Verification items for the finished model (mm, model axes). A direction names the side the tool comes from. Give positions to 0.01 mm unless a question says otherwise; leave off trailing zeros. Loops run counter-clockwise (first coordinate to the right, second up) from the corner with the lowest first, then second, coordinate; pieces in that order, holes last. Notation, with made-up numbers: (77, -23.75) -> (108, -23.75) arc R33 cw to (108, 6.25) -> close; hole circle Ø5 at (-40, 23.5). An arc over 180 degrees is marked (long way). Answer in a Markdown table with one row per item. Add a question column.
Q1. Gauge pin test, flat ends, axial feed: P1, Ø1, axis at x = -440.5, y = -16, coming from the -Z side; P2, Ø4, axis at x = -154.5, y = -15.5, coming from the +Z side. Record the tip position at first contact, or that the pin passes through.
Q2. Material ranges on probe 1 along X at (y, z) = (-17.25, 167) (3 decimals); probe 2 along Z at (x, y) = (-696.5, -17.25); probe 3 along X at (y, z) = (-10.5, 149), recorded low to high.
Q3. Section check D-D on z = 49.5. Enter the section's corners in (x, y).
Q4. Section check A-A on z = 178. Enter the section's corners in (x, y) (3 decimals), and give its area (3 significant figures).
Q5. Section check B-B on y = -15.25. Enter the section's corners in (x, z) (3 decimals).
Q6. Release check for a two-part mould opening along X. For faces 1 (the face through (-422, 0, 103)), 2 (the face through (-92.968, -9.392, 147.338)), 3 (the face through (-831.85, -9, 103)) record: pulls with the +X half, pulls with the -X half, needs draft (parallel to the pull), parting line crosses it, or undercut.
Q7. Set-up check for faces 4 (the face through (-746.125, -9, 22)), 5 (the face through (-793, -9, 0)), 6 (the face through (-412, -9, 139.7)): record each of +Z, -Z, +X, -X, +Y, -Y from which the full face is reachable in a straight line by a thin tool's end or side.
Q8. Section check C-C on x = -547. Enter the section's corners in (y, z), and give its area (3 significant figures).
```python
from build123d import *

# Parameters (mm, degrees)
F1_DEPTH = 19.05


with BuildPart() as f1:
    # F0 (on Front) → F1 (new body)
    with BuildSketch(Plane.XZ):
        with BuildLine():
            Line((-752.475, 203.2), (-831.85, 203.2))
            Line((-831.85, 203.2), (-831.85, 0))
            Line((-831.85, 0), (-752.475, 0))
            ThreePointArc((-752.475, 0), (-747.984872, 1.859872), (-746.125, 6.35))
            Line((-746.125, 6.35), (-746.125, 38.1))
            ThreePointArc((-746.125, 38.1), (-738.685512, 56.060512), (-720.725, 63.5))
            Line((-720.725, 63.5), (-111.125, 63.5))
            ThreePointArc((-111.125, 63.5), (-93.164488, 56.060512), (-85.725, 38.1))
            Line((-85.725, 38.1), (-85.725, 6.35))
            ThreePointArc((-85.725, 6.35), (-83.865128, 1.859872), (-79.375, 0))
            Line((-79.375, 0), (0, 0))
            Line((0, 0), (0, 203.2))
            Line((0, 203.2), (-79.375, 203.2))
            ThreePointArc((-79.375, 203.2), (-83.865128, 201.340128), (-85.725, 196.85))
            Line((-85.725, 196.85), (-85.725, 165.1))
            ThreePointArc((-85.725, 165.1), (-93.164488, 147.139488), (-111.125, 139.7))
            Line((-111.125, 139.7), (-720.725, 139.7))
            ThreePointArc((-720.725, 139.7), (-738.685512, 147.139488), (-746.125, 165.1))
            Line((-746.125, 165.1), (-746.125, 196.85))
            ThreePointArc((-746.125, 196.85), (-747.984872, 201.340128), (-752.475, 203.2))
        make_face()
    extrude(amount=F1_DEPTH)


solid = f1.part
```
Taken from the geometry:
| question | item | result |
|---|---|---|
| 1 | P1 | stops at z = 63.5 |
| 1 | P2 | stops at z = 139.7 |
| 2 | probe 1 | x = -831.85 to -746.125, -85.725 to 0 |
| 2 | probe 2 | z = 63.5 to 139.7 |
| 2 | probe 3 | x = -831.85 to -740.37, -91.48 to 0 |
| 3 | outline | (-831.85, -19.05) -> (-743.42, -19.05) -> (-743.42, 0) -> (-831.85, 0) -> close; (-88.43, -19.05) -> (0, -19.05) -> (0, 0) -> (-88.43, 0) -> close |
| 4 | outline | (-831.85, -19.05) -> (-746.125, -19.05) -> (-746.125, 0) -> (-831.85, 0) -> close; (-85.725, -19.05) -> (0, -19.05) -> (0, 0) -> (-85.725, 0) -> close |
| 4 | area | 3,270 mm² |
| 5 | outline | (-831.85, 0) -> (-752.475, 0) arc R6.35 ccw to (-746.125, 6.35) -> (-746.125, 38.1) arc R25.4 cw to (-720.725, 63.5) -> (-111.125, 63.5) arc R25.4 cw to (-85.725, 38.1) -> (-85.725, 6.35) arc R6.35 ccw to (-79.375, 0) -> (0, 0) -> (0, 203.2) -> (-79.375, 203.2) arc R6.35 ccw to (-85.725, 196.85) -> (-85.725, 165.1) arc R25.4 cw to (-111.125, 139.7) -> (-720.725, 139.7) arc R25.4 cw to (-746.125, 165.1) -> (-746.125, 196.85) arc R6.35 ccw to (-752.475, 203.2) -> (-831.85, 203.2) -> close |
| 6 | face 1 | needs draft |
| 6 | face 2 | undercut |
| 6 | face 3 | pulls with the -X half |
| 7 | face 4 | -Z, +Y, -Y |
| 7 | face 5 | -Z, +X, -X, +Y, -Y |
| 7 | face 6 | +Z, +Y, -Y |
| 8 | outline | (-19.05, 63.5) -> (0, 63.5) -> (0, 139.7) -> (-19.05, 139.7) -> close |
| 8 | area | 1,450 mm² |
